Part print with two shaded views. Sizes in mm from the minimum x, y, z corner. A direction names the side the tool comes from. Coordinates: 2 decimals unless noted, no trailing zeros. Order: outer loops, then holes, each group sorted by start corner. A loop starts at its lowest first (then second) coordinate and runs counter-clockwise, first axis right, second up.
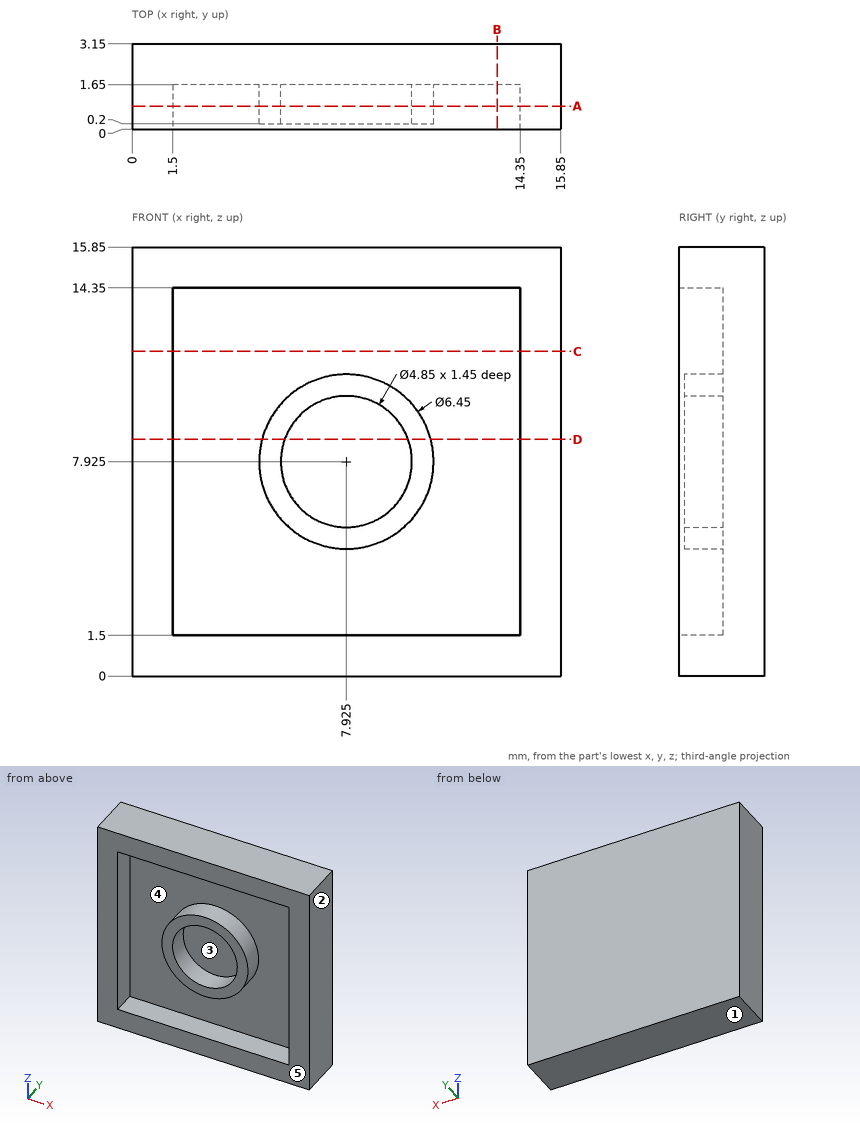
Q1. Which spindle directions (+Z, -Z, +X, -X, +Y, -Y) get a long thin tool onto all of the face, cutting with end or side? Do the marked faces 4 and 5. Say none if no direction does.
Results list:
face 4: -Y
face 5: +Z, -Z, +X, -X, -Y
Q2. Cut at D-D on z = 8.75. Write the cut outline in (x, y).
Results list:
outline: (0, 0) - (1.5, 0) - (1.5, 1.65) - (4.81, 1.65) - (4.81, 0.2) - (5.64, 0.2) - (5.64, 1.65) - (10.21, 1.65) - (10.21, 0.2) - (11.04, 0.2) - (11.04, 1.65) - (14.35, 1.65) - (14.35, 0) - (15.85, 0) - (15.85, 3.15) - (0, 3.15) - close
Q3. Cut at B-B on x = 13.5. Write the cut outline in (y, z), and give its area (3 significant figures).
Results list:
outline: (0, 0) - (3.15, 0) - (3.15, 15.85) - (0, 15.85) - (0, 14.35) - (1.65, 14.35) - (1.65, 1.5) - (0, 1.5) - close
area: 28.7 mm2
Q4. Cut at A-A on y = 0.85. Write the cut outline in (x, z) (3 decimals), and give its area (3 significant figures).
Results list:
outline: (0, 0) - (15.85, 0) - (15.85, 15.85) - (0, 15.85) - close; circle Ø6.45 at (7.925, 7.925); hole (1.5, 1.5) - (14.35, 1.5) - (14.35, 14.35) - (1.5, 14.35) - close; hole circle Ø4.85 at (7.925, 7.925)
area: 100 mm2
Q5. Wall check: line 1 along X through (y, z) = (1.5, 3.25); line 2 along Z through (x, y) = (9, 1.35); line 3 along Z through (x, y) = (10, 1.55). Give the ranges that are in metal, low to high.
Results list:
line 1: x = 0 to 1.5, 14.35 to 15.85
line 2: z = 0 to 1.5, 4.88 to 5.75, 10.1 to 10.97, 14.35 to 15.85
line 3: z = 0 to 1.5, 5.46 to 6.67, 9.18 to 10.39, 14.35 to 15.85
Q6. Cut at C-C on z = 12. Write the cut outline in (x, y), and give its area (3 significant figures).
Results list:
outline: (0, 0) - (1.5, 0) - (1.5, 1.65) - (14.35, 1.65) - (14.35, 0) - (15.85, 0) - (15.85, 3.15) - (0, 3.15) - close
area: 28.7 mm2
Q7. Pin check, flat tips, straight feed: pin 1 Ø1.5 at (y, z) = (2, 5.5) entering from -X; pin 2 Ø1.9 at (x, z) = (9, 9) entering from -Y. Stop position of each tip, or through.
Results list:
pin 1: stops at x = 0
pin 2: stops at y = 0.2
Q8. Mould opens along Z. For the marked faces 1, 2 and 3 say: pulls with the +Z half, pulls with the -Z half, needs draft (parallel to the pull), parting line crosses it, or undercut.
Results list:
face 1: pulls with the -Z half
face 2: needs draft
face 3: undercut
